from build123d import *

# Parameters (mm, degrees)
SKETCH_1_W                  = 40
SKETCH_1_H                  = 20
EXTRUDE_1_DEPTH             = 2
HOLE_WIZARD_M3_1_AT_2_COUNT = 2
HOLE_WIZARD_M3_1_AT_2_PITCH = 27


with BuildPart() as part:
    # 草圖1 → 填料-伸長1 (new body)
    with BuildSketch(Plane.XY):
        Rectangle(SKETCH_1_W, SKETCH_1_H)
    extrude(amount=EXTRUDE_1_DEPTH)

    # 草圖2 → M3 平錐坑頭螺釘的錐孔1 (revolve, cut)
    with BuildSketch(Plane(origin=(-13.5, 5, 2), x_dir=(0, -1, 0), z_dir=(1, 0, 0))):
        Polygon((0, 0), (0, 2), (1.7, 2), (1.7, 1.45), (3.15, 0), align=None)
    hole_wizard_m3_1 = revolve(axis=Axis((-13.5, 5, 8.35), (0, 0, -1)), mode=Mode.SUBTRACT)

    # M3 平錐坑頭螺釘的錐孔1 at 2: M3 平錐坑頭螺釘的錐孔1 ×2
    with Locations(*[(i * HOLE_WIZARD_M3_1_AT_2_PITCH, 0, 0) for i in range(1, HOLE_WIZARD_M3_1_AT_2_COUNT)]):
        add(hole_wizard_m3_1, mode=Mode.SUBTRACT)


solid = part.part
Here's how the part is built. I have some questions about the finished solid (model axes, mm). Give positions to 0.01 mm unless a question says otherwise; leave off trailing zeros. Order: outer loops, then holes, each group sorted by start corner. A loop starts at its lowest first (then second) coordinate and runs counter-clockwise, first axis right, second up. Notation, with made-up numbers: (-15, 25.5) -> (-2, 25.5) arc R19 ccw to (-2, 57.5) -> close; hole circle Ø4 at (38.25, 60). An arc over 180 degrees is marked (long way). Use a Markdown table: item, result. Add a question column.
Item 1: If we mould it in two halves opening along X, with no side actions, what happens to faces 1 (the face through (0, 0, 2)), 2 (the face through (-14.933, 4.086, 0.279)), 3 (the face through (-20, 0, 1))? For each: pulls with the +X half, pulls with the -X half, needs draft (parallel to the pull), parting line crosses it, or undercut.
Item 2: Imagine slicing it at B-B on x = -13.5. Please give me the cut outline in (y, z), plus the area to 3 significant figures.
Item 3: Will these pins go through, and if not, where does the flat tip stop? pin 1 (3 mm diameter, centred on x = -13.5, y = 5, fed in from -Z); pin 2 (4.5 mm diameter, centred on x = 13.5, y = 5, fed in from +Z).
Item 4: I need wall thicknesses on line 1 (X direction, y = 5, z = 0.35); line 2 (Y direction, x = 13.5, z = 0.2); line 3 (X direction, y = 5.5, z = 1.5). Which ranges of each line are inside material? Lowest first, please.
Item 5: Imagine slicing it at C-C on z = 1.65. Please give me the cut outline in (x, y).
Item 6: Imagine slicing it at A-A on y = 5. Please give me the cut outline in (x, z), plus the area to 3 significant figures.
Data:
| question | item | result |
|---|---|---|
| 1 | face 1 | needs draft |
| 1 | face 2 | undercut |
| 1 | face 3 | pulls with the -X half |
| 2 | outline | (-10, 0) -> (3.3, 0) -> (3.3, 0.55) -> (1.85, 2) -> (-10, 2) -> close; (6.7, 0) -> (10, 0) -> (10, 2) -> (8.15, 2) -> (6.7, 0.55) -> close |
| 2 | area | 31.1 mm² |
| 3 | pin 1 | passes through |
| 3 | pin 2 | stops at z = 1.1 |
| 4 | line 1 | x = -20 to -15.2, -11.8 to 11.8, 15.2 to 20 |
| 4 | line 2 | y = -10 to 3.3, 6.7 to 10 |
| 4 | line 3 | x = -20 to -16.1, -10.9 to 10.9, 16.1 to 20 |
| 5 | outline | (-20, -10) -> (20, -10) -> (20, 10) -> (-20, 10) -> close; hole circle Ø5.6 at (-13.5, 5); hole circle Ø5.6 at (13.5, 5) |
| 6 | outline | (-20, 0) -> (-15.2, 0) -> (-15.2, 0.55) -> (-16.65, 2) -> (-20, 2) -> close; (-11.8, 0) -> (11.8, 0) -> (11.8, 0.55) -> (10.35, 2) -> (-10.35, 2) -> (-11.8, 0.55) -> close; (15.2, 0) -> (20, 0) -> (20, 2) -> (16.65, 2) -> (15.2, 0.55) -> close |
| 6 | area | 62.2 mm² |
